Read the model definition and answer for the solid it produces. Units are mm, in the model's axes. A direction names the side the tool comes from. Round coordinates to 2 decimals unless told otherwise and drop trailing zeros. Loops run counter-clockwise (first coordinate to the right, second up) from the corner with the lowest first, then second, coordinate; pieces in that order, holes last. Notation, with made-up numbers: (26, 30.25) - (36, 30.25) arc R24 ccw to (36, 62.25) - close; hole circle Ø2 at (39, 83.5). An arc over 180 degrees is marked (long way). Use one line per item in the form item = value. Start each with the question number.
```python
from build123d import *

# Parameters (mm, degrees)
SKETCH1_W           = 84.836
SKETCH1_H           = 69.342
BASE_FLANGE1_DEPTH  = 4.826
SKETCH6_R           = 2.54
CUT_EXTRUDE1_DEPTH  = 10
FILLET1_R           = 2.6
SKETCH11_W          = 59.436
SKETCH11_H          = 3.175
SKETCH11_W_2        = 5.08
SKETCH11_H_2        = 43.942
SKETCH11_W_3        = 2.794
BOSS_EXTRUDE1_DEPTH = 6.35
SKETCH12_W          = 59.436
SKETCH12_H          = 53.848
CUT_EXTRUDE5_DEPTH  = 56.151495583


# Sheet-metal steps are written as plain solids
with BuildPart() as part:
    # Sketch1 → Base-Flange1 (new body)
    with BuildSketch(Plane.XY):
        Rectangle(SKETCH1_W, SKETCH1_H)
    extrude(amount=-BASE_FLANGE1_DEPTH)

    # Sketch6 → Cut-Extrude1 (cut)
    with BuildSketch(Plane.XY):
        with Locations((-37.465, 29.718)):
            Circle(SKETCH6_R)
        with Locations(Location((-37.465, -29.718, 0), (0, 0, 180))):
            Circle(SKETCH6_R)
        with Locations((37.465, -29.718)):
            Circle(SKETCH6_R)
        with Locations(Location((37.465, 29.718, 0), (0, 0, 180))):
            Circle(SKETCH6_R)
    extrude(amount=-CUT_EXTRUDE1_DEPTH, mode=Mode.SUBTRACT)

    # Fillet1
    fillet1_edges = [part.edges().sort_by_distance(p)[0] for p in [
        (-42.418, 34.671, -2.413),
        (42.418, 34.671, -2.413),
        (42.418, -34.671, -2.413),
        (-42.418, -34.671, -2.413),
    ]]
    fillet(fillet1_edges, radius=FILLET1_R)

    # Sketch11 → Boss-Extrude1 (add)
    with BuildSketch(Plane(origin=(0, 0, -4.826), x_dir=(-1, 0, 0), z_dir=(0, 0, -1))):
        with Locations((0, 28.5115)):
            Rectangle(SKETCH11_W, SKETCH11_H)
        with Locations((35.306, 0)):
            Rectangle(SKETCH11_W_2, SKETCH11_H_2)
        with Locations((0, -28.5115)):
            Rectangle(SKETCH11_W, SKETCH11_H)
        with Locations((-36.449, 0)):
            Rectangle(SKETCH11_W_3, SKETCH11_H_2)
    extrude(amount=BOSS_EXTRUDE1_DEPTH)

    # Sketch12 → Cut-Extrude5 (cut, through all)
    with BuildSketch(Plane(origin=(0, 0, -4.826), x_dir=(-1, 0, 0), z_dir=(0, 0, -1))):
        Rectangle(SKETCH12_W, SKETCH12_H)
    extrude(amount=-CUT_EXTRUDE5_DEPTH, mode=Mode.SUBTRACT)


solid = part.part
```
1) Flat-ended cylindrical pins translate along their axes: pin 1 (4 mm diameter, centred on x = -29, z = -8.5, fed in from +Y); pin 2 (2.5 mm diameter, centred on x = -36, z = -7.5, fed in from +Y); pin 3 (3 mm diameter, centred on y = -10.5, z = -8, fed in from -X); pin 4 (3.5 mm diameter, centred on y = -29, z = -6.5, fed in from -X). Find the tip coordinate at first contact, or state that the pin passes through.
2) A cutting plane is placed at D-D on z = -3. Write down the section's boundary in (x, y) (3 decimals), plus the area to 3 significant figures.
3) Determine the mould class of faces 1 (the cylindrical face through (-35.04, 30.48, -2.38)), 2 (the flat face through (0, -28, -11.176)), 3 (the cylindrical face through (-41.677, 33.889, -2.447)) for opening direction X: +X half, -X half, draft (parallel to the pull), parting line (faces both ways), or undercut.
4) A cutting plane is placed at A-A on y = 25.5. Write down the section's boundary in (x, z).
5) A cutting plane is placed at B-B on z = -8.75. Write down the section's boundary in (x, y), plus the area to 3 significant figures.
6) Straight lines are drawn through the part: line 1 (Y direction, x = -2.5, z = -8.75); line 2 (Y direction, x = -2, z = -0.75); line 3 (X direction, y = -18, z = -7.5). For each, find the intervals that lie inside material, in ascending order. Write a range as from..to.
7) A cutting plane is placed at C-C on x = 13.5. Write down the section's boundary in (y, z), plus the area to 3 significant figures.
8) For faces 4 (the flat face through (0, 30.099, -8)), 5 (the flat face through (-37.846, 0, -8)), 6 (the flat face through (0, -26.924, -6)), 7 (the flat face through (29.718, 28, -8)), determine the directions among +Z, -Z, +X, -X, +Y, -Y from which every point of the face is accessible in a straight line to the end or side of a thin tool.
Checks:
q1.pin_1 = 30.1
q1.pin_2 = 21.97
q1.pin_3 = -37.85
q1.pin_4 = -42.42
q2.outline = (-42.418, -32.071) arc R2.6 ccw to (-39.818, -34.671) - (39.818, -34.671) arc R2.6 ccw to (42.418, -32.071) - (42.418, 32.071) arc R2.6 ccw to (39.818, 34.671) - (-39.818, 34.671) arc R2.6 ccw to (-42.418, 32.071) - close; hole circle Ø5.08 at (-37.465, -29.718); hole circle Ø5.08 at (-37.465, 29.718); hole (-29.718, -26.924) - (29.718, -26.924) - (29.718, 26.924) - (-29.718, 26.924) - close; hole circle Ø5.08 at (37.465, -29.718); hole circle Ø5.08 at (37.465, 29.718)
q2.area = 2,600 mm²
q3.face_1 = undercut
q3.face_2 = draft
q3.face_3 = -X half
q4.outline = (-42.42, -4.83) - (-29.72, -4.83) - (-29.72, 0) - (-42.42, 0) - close; (29.72, -4.83) - (42.42, -4.83) - (42.42, 0) - (29.72, 0) - close
q5.outline = (-37.85, -21.97) - (-32.77, -21.97) - (-32.77, 21.97) - (-37.85, 21.97) - close; (-29.72, -30.1) - (29.72, -30.1) - (29.72, -26.92) - (-29.72, -26.92) - close; (-29.72, 26.92) - (29.72, 26.92) - (29.72, 30.1) - (-29.72, 30.1) - close; (35.05, -21.97) - (37.85, -21.97) - (37.85, 21.97) - (35.05, 21.97) - close
q5.area = 723 mm²
q6.line_1 = -30.1..-26.92, 26.92..30.1
q6.line_2 = -34.67..-26.92, 26.92..34.67
q6.line_3 = -37.85..-32.77, 35.05..37.85
q7.outline = (-34.67, -4.83) - (-30.1, -4.83) - (-30.1, -11.18) - (-26.92, -11.18) - (-26.92, 0) - (-34.67, 0) - close; (26.92, -11.18) - (30.1, -11.18) - (30.1, -4.83) - (34.67, -4.83) - (34.67, 0) - (26.92, 0) - close
q7.area = 115 mm²
q8.face_4 = -Z, +X, -X, +Y
q8.face_5 = -Z, -X, +Y, -Y
q8.face_6 = +Z, -Z
q8.face_7 = -Z, +X, +Y, -Y
